Design review of the part built by this model. Coordinates are the model's own, in mm. Round coordinates to 2 decimals unless told otherwise and drop trailing zeros. Loops run counter-clockwise (first coordinate to the right, second up) from the corner with the lowest first, then second, coordinate; pieces in that order, holes last. Notation, with made-up numbers: (41.5, 27.5) -> (72.5, 27.5) arc R24 ccw to (72.5, 46.5) -> close; hole circle Ø1 at (15, -14). An arc over 180 degrees is marked (long way). Answer as CSV lines item,"result". Start each with the question number.
(1) Take a section at C-C, the plane y = 25.5. Write out the cut boundary in (x, z), and give its area (3 significant figures).
(2) Take a section at B-B, the plane x = -11.5. Write out the cut boundary in (y, z).
(3) To check wall thickness, follow line 1 (Y direction, x = 2, z = 0.2); line 2 (Y direction, x = 0, z = 1.25); line 3 (Y direction, x = -2, z = 1.8). State the ranges of each line that lie inside material, in increasing order. Write a range as from..to.
(4) For P1, Ø0.9, axis at y = -4.5, z = 1, coming from the -X side; P2, Ø0.9, axis at x = 11.5, z = 2, coming from the +Y side; P3, Ø4, axis at x = 3.5, y = 13.5, coming from the -Z side; P4, Ø0.9, axis at y = 4.5, z = 2, coming from the +X side, all flat-tipped, find the tip position at first contact; note any pin that passes through.
(5) Take a section at A-A, the plane y = 0. Write out the cut boundary in (x, z).
(6) Take a section at D-D, the plane x = 4. Write out the cut boundary in (y, z).
from build123d import *

# Parameters (mm, degrees)
F0_R      = 30.135624
F1_DEPTH  = 3
F2_R      = 1.590818
F3_DEPTH  = 25
F5_DEPTH  = 25
F6_W      = 3.730636
F6_H      = 14.922548
F7_DEPTH  = 25
F8_W      = 14.922549
F8_H      = 3.544105
F9_DEPTH  = 25
F10_W     = 3.357574
F10_H     = 14.176421
F11_DEPTH = 25
F12_W     = 15.295613
F12_H     = 3.730637
F13_DEPTH = 25
F14_W     = 17.537619
F14_H     = 2.187502
F14_H_2   = 2.134302
F15_DEPTH = 25


with BuildPart() as f1:
    # F0 (on Top) → F1 (new body)
    with BuildSketch(Plane.XY):
        Circle(F0_R)
    extrude(amount=F1_DEPTH)

    # F2 (on face) → F3 (cut)
    with BuildSketch(Plane.XY.offset(3)):
        Circle(F2_R)
    extrude(amount=-F3_DEPTH, mode=Mode.SUBTRACT)

    # F4 (on face) → F5 (cut)
    with BuildSketch(Plane.XY.offset(3)):
        Polygon((0.042525, 5.293039), (9.073219, 21.08197), (-9.115743, 21.008315), align=None)
        Polygon((0.042525, -25.99019), (9.073219, -10.201259), (-9.115743, -10.274914), align=None)
    extrude(amount=-F5_DEPTH, mode=Mode.SUBTRACT)

    # F6 (on face) → F7 (cut)
    with BuildSketch(Plane.XY.offset(3)):
        with Locations((-17.842693, 0.09647)):
            Rectangle(F6_W, F6_H)
    extrude(amount=-F7_DEPTH, mode=Mode.SUBTRACT)

    # F8 (on face) → F9 (cut)
    with BuildSketch(Plane.XY.offset(3)):
        with Locations((-18.029225, 0.189735)):
            Rectangle(F8_W, F8_H)
    extrude(amount=-F9_DEPTH, mode=Mode.SUBTRACT)

    # F10 (on face) → F11 (cut)
    with BuildSketch(Plane.XY.offset(3)):
        with Locations((17.78489, 0.469533)):
            Rectangle(F10_W, F10_H)
    extrude(amount=-F11_DEPTH, mode=Mode.SUBTRACT)

    # F12 (on face) → F13 (cut)
    with BuildSketch(Plane.XY.offset(3)):
        with Locations((17.411827, 0.096469)):
            Rectangle(F12_W, F12_H)
    extrude(amount=-F13_DEPTH, mode=Mode.SUBTRACT)

    # F14 (on face) → F15 (cut)
    with BuildSketch(Plane.XY.offset(3)):
        with Locations((-0.346934, 25.265625)):
            Rectangle(F14_W, F14_H)
        with Locations((-0.346934, -5.551526)):
            Rectangle(F14_W, F14_H_2)
    extrude(amount=-F15_DEPTH, mode=Mode.SUBTRACT)


solid = f1.part
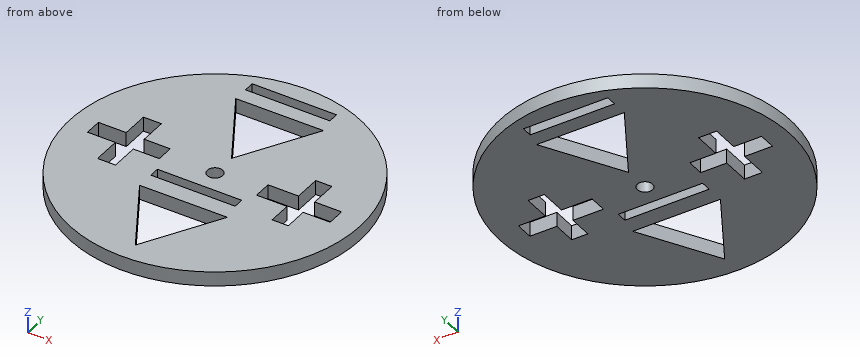
The answers:
1,outline,"(-16.06, 0) -> (-9.12, 0) -> (-9.12, 3) -> (-16.06, 3) -> close; (8.42, 0) -> (16.06, 0) -> (16.06, 3) -> (8.42, 3) -> close"
1,area,"43.7 mm²"
2,outline,"(-27.86, 0) -> (-1.58, 0) -> (-1.58, 3) -> (-27.86, 3) -> close; (1.96, 0) -> (27.86, 0) -> (27.86, 3) -> (1.96, 3) -> close"
3,line 1,"-30.07..-22.57, -10.23..-6.62, -4.48..8.72, 21.05..24.17, 26.36..30.07"
3,line 2,"-30.14..-25.92, -10.24..-6.62, -4.48..-1.59, 1.59..5.37, 21.05..24.17, 26.36..30.14"
3,line 3,"-30.07..-22.49, -10.25..-6.62, -4.48..8.8, 21.04..24.17, 26.36..30.07"
4,P1,"x = -29.86"
4,P2,"y = 28.04"
4,P3,"z = 0"
4,P4,"x = 29.86"
5,outline,"(-30.14, 0) -> (-25.49, 0) -> (-25.49, 3) -> (-30.14, 3) -> close; (-10.57, 0) -> (-1.59, 0) -> (-1.59, 3) -> (-10.57, 3) -> close; (1.59, 0) -> (9.76, 0) -> (9.76, 3) -> (1.59, 3) -> close; (25.06, 0) -> (30.14, 0) -> (30.14, 3) -> (25.06, 3) -> close"
6,outline,"(-29.87, 0) -> (-19.07, 0) -> (-19.07, 3) -> (-29.87, 3) -> close; (-10.22, 0) -> (-6.62, 0) -> (-6.62, 3) -> (-10.22, 3) -> close; (-4.48, 0) -> (12.21, 0) -> (12.21, 3) -> (-4.48, 3) -> close; (21.06, 0) -> (24.17, 0) -> (24.17, 3) -> (21.06, 3) -> close; (26.36, 0) -> (29.87, 0) -> (29.87, 3) -> (26.36, 3) -> close"
